Input: dimensioned drawing with shaded views. Units: mm. Origin: part minimum x, y, z. Coordinates: 2 decimals unless noted, no trailing zeros. Loops run counter-clockwise (first coordinate to the right, second up) from the corner with the lowest first, then second, coordinate; pieces in that order, holes last.
Item 1: Section B-B on x = 5.08. Return loops of the section in (y, z), and give its area (3 significant figures).
Item 2: Section D-D on z = 63.08. Return loops of the section in (x, y).
Item 3: Section C-C on y = 4.1. Return loops of the section in (x, z).
Item 4: Section A-A on z = 5.08. Return loops of the section in (x, y).
Item 5: Ray query, line 1 along X through (y, z) = (0.45, 5.08); line 2 along X through (y, z) = (4.1, 63.5); line 3 along Z through (x, y) = (30.5, 2.8). Return the intervals inside material, ascending.
Item 6: Contact query for flat-ended pins moving along their axis: P1, Ø1.8, axis at x = 4.5, z = 120.5, coming from the +Y side; P2, Ø1.5, axis at x = 12.5, y = 2, coming from the -Z side; P3, Ø2, axis at y = 3, z = 35.5, coming from the -X side. Output: stop coordinate, or through.
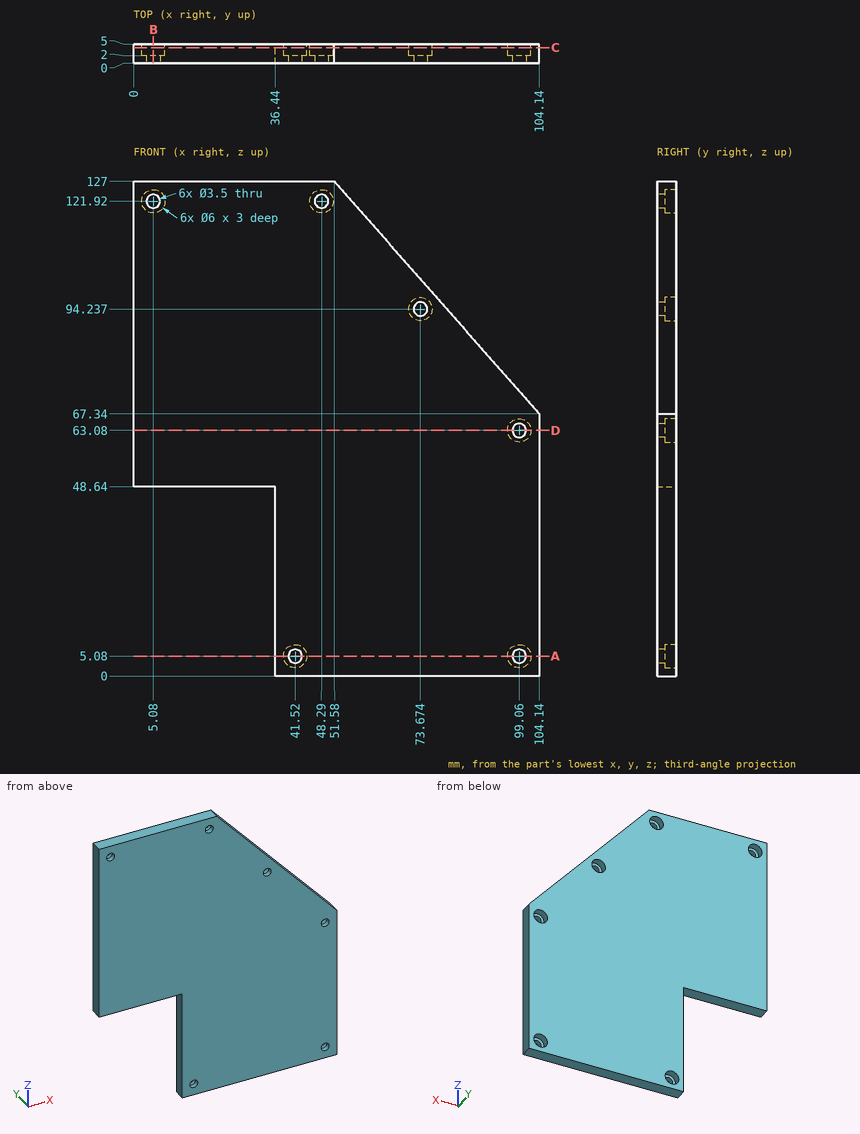
Results found:
1. outline: (0, 48.64) - (5, 48.64) - (5, 118.92) - (2, 118.92) - (2, 120.17) - (0, 120.17) - close; (0, 123.67) - (2, 123.67) - (2, 124.92) - (5, 124.92) - (5, 127) - (0, 127) - close
1. area: 367 mm2
2. outline: (0, 0) - (97.31, 0) - (97.31, 2) - (96.06, 2) - (96.06, 5) - (0, 5) - close; (100.81, 0) - (104.14, 0) - (104.14, 5) - (102.06, 5) - (102.06, 2) - (100.81, 2) - close
3. outline: (0, 48.64) - (36.44, 48.64) - (36.44, 0) - (104.14, 0) - (104.14, 67.34) - (51.58, 127) - (0, 127) - close; hole circle Ø6 at (5.08, 121.92); hole circle Ø6 at (41.52, 5.08); hole circle Ø6 at (48.29, 121.92); hole circle Ø6 at (73.67, 94.24); hole circle Ø6 at (99.06, 5.08); hole circle Ø6 at (99.06, 63.08)
4. outline: (36.44, 0) - (39.77, 0) - (39.77, 2) - (38.52, 2) - (38.52, 5) - (36.44, 5) - close; (43.27, 0) - (97.31, 0) - (97.31, 2) - (96.06, 2) - (96.06, 5) - (44.52, 5) - (44.52, 2) - (43.27, 2) - close; (100.81, 0) - (104.14, 0) - (104.14, 5) - (102.06, 5) - (102.06, 2) - (100.81, 2) - close
5. line 1: x = 36.44 to 39.77, 43.27 to 97.31, 100.81 to 104.14
5. line 2: x = 0 to 96.09, 102.03 to 104.14
5. line 3: z = 48.64 to 127
6. P1: stops at y = 2
6. P2: stops at z = 48.64
6. P3: stops at x = 36.44
